Part model, mm, in its own coordinate system. A direction names the side the tool comes from. Round coordinates to 2 decimals unless told otherwise and drop trailing zeros. Write each loop counter-clockwise with the first axis right and the second up, starting at its lowest first coordinate (ties: lowest second). Pieces come first, ordered by that corner, then holes.
```python
from build123d import *

# Parameters (mm, degrees)
F0_R     = 15
F1_DEPTH = 80.5
F2_W     = 45
F2_H     = 11.5
F2_W_2   = 39
F3_DEPTH = 15
F4_R     = 10
F5_R     = 6
F6_DEPTH = 3.5


with BuildPart() as f1:
    # F0 (on Right) → F1 (new body, symmetric)
    with BuildSketch(Plane.YZ):
        Circle(F0_R)
    extrude(amount=F1_DEPTH, both=True)

    # F2 (on Front) → F3 (cut, symmetric)
    with BuildSketch(Plane.XZ):
        with Locations((-58, 9.25)):
            Rectangle(F2_W, F2_H)
        with Locations((-58, -9.25)):
            Rectangle(F2_W, F2_H)
        with Locations((61, 9.25)):
            Rectangle(F2_W_2, F2_H)
        with Locations((61, -9.25)):
            Rectangle(F2_W_2, F2_H)
    extrude(amount=F3_DEPTH, both=True, mode=Mode.SUBTRACT)

    # F4
    f4_edges = [f1.edges().sort_by_distance(p)[0] for p in [
        (41.5, 0, 3.5),
        (-35.5, 0, 3.5),
        (41.5, 0, -3.5),
        (-35.5, 0, -3.5),
    ]]
    fillet(f4_edges, radius=F4_R)

    # F5 (on Top) → F6 (cut, symmetric)
    with BuildSketch(Plane.XY):
        with Locations((-65.5, 0)):
            Circle(F5_R)
        with BuildLine():
            Line((67.5, 6), (63.5, 6))
            ThreePointArc((63.5, 6), (57.5, 0), (63.5, -6))
            Line((63.5, -6), (67.5, -6))
            ThreePointArc((67.5, -6), (73.5, 0), (67.5, 6))
        make_face()
    extrude(amount=F6_DEPTH, both=True, mode=Mode.SUBTRACT)


solid = f1.part
```
Q1. Cut at D-D on x = 24.5. Write the cut outline in (y, z), plus the area to 3 significant figures.
Values follow:
outline: circle Ø30 at (0, 0)
area: 707 mm2
Q2. Cut at B-B on z = 0. Write the cut outline in (x, y), plus the area to 3 significant figures.
Values follow:
outline: (-80.5, -15) - (80.5, -15) - (80.5, 15) - (-80.5, 15) - close; hole circle Ø12 at (-65.5, 0); hole (63.5, -6) - (67.5, -6) arc R6 ccw to (67.5, 6) - (63.5, 6) arc R6 ccw to start
area: 4,560 mm2
Q3. Drop flat-ended pins along their axis: pin 1 (1.5 mm diameter, centred on x = -53.5, y = -0.5, fed in from +Z); pin 2 (11 mm diameter, centred on x = -65.5, y = 0, fed in from +Z); pin 3 (1.2 mm diameter, centred on y = 2, z = -14.5, fed in from +X); pin 4 (4 mm diameter, centred on x = -7, z = 10.5, fed in from -Y). Give the stop position or say it passes through.
Values follow:
pin 1: stops at z = 3.5
pin 2: passes through
pin 3: stops at x = 41.5
pin 4: stops at y = -12.36
Q4. Wall check: L1, parallel to X at y = -2.5, z = 1; L2, parallel to Z at x = 63, y = 9.5; L3, parallel to Y at x = 0.5, z = -6.5. Give the ranges that are in metal, low to high.
Values follow:
L1: x = -80.5 to -70.95, -60.05 to 58.05, 72.95 to 80.5
L2: z = -3.5 to 3.5
L3: y = -13.52 to 13.52
Q5. Cut at A-A on x = -65.5. Write the cut outline in (y, z), plus the area to 3 significant figures.
Values follow:
outline: (-14.59, -3.5) - (-6, -3.5) - (-6, 3.5) - (-14.59, 3.5) arc R15 ccw to start; (6, -3.5) - (14.59, -3.5) arc R15 ccw to (14.59, 3.5) - (6, 3.5) - close
area: 124 mm2
Q6. Which spindle directions (+Z, -Z, +X, -X, +Y, -Y) get a long thin tool onto all of the face, cutting with end or side? Do faces 5 (the cylindrical face through (73.5, -0.1, 0)), 6 (the flat face through (66, 7, 3.5)), 7 (the flat face through (-59, 0, 3.5)). Say none if no direction does.
Values follow:
face 5: +Z, -Z
face 6: +Z, +X, +Y, -Y
face 7: +Z, -X, +Y, -Y
Q7. Mould opens along X. For faces 1 (the flat face through (65, -6, 0)), 2 (the cylindrical face through (-38.35, -0.2, 6.51)), 3 (the cylindrical face through (-71.494, 0.264, -0.049)), 4 (the flat face through (-59, 0, -3.5)) say: +X half, -X half, draft (parallel to the pull), parting line (faces both ways), or undercut.
Values follow:
face 1: undercut
face 2: -X half
face 3: undercut
face 4: draft
Q8. Cut at C-C on y = -12. Write the cut outline in (x, z), plus the area to 3 significant figures.
Values follow:
outline: (-80.5, -3.5) - (-45.5, -3.5) arc R10 cw to (-36.57, -9) - (42.57, -9) arc R10 cw to (51.5, -3.5) - (80.5, -3.5) - (80.5, 3.5) - (51.5, 3.5) arc R10 cw to (42.57, 9) - (-36.57, 9) arc R10 cw to (-45.5, 3.5) - (-80.5, 3.5) - close
area: 2,050 mm2
